Geometry check sheet. Reference: the model listing, model coordinates, mm. Round coordinates to 2 decimals unless told otherwise and drop trailing zeros. Loops run counter-clockwise (first coordinate to the right, second up) from the corner with the lowest first, then second, coordinate; pieces in that order, holes last. Notation, with made-up numbers: (74, 75.5) - (105, 75.5) arc R16 ccw to (105, 91.5) - close; hole circle Ø5 at (83.5, 35.5). An arc over 180 degrees is marked (long way). Answer in a Markdown table with one row per item. Add a question column.
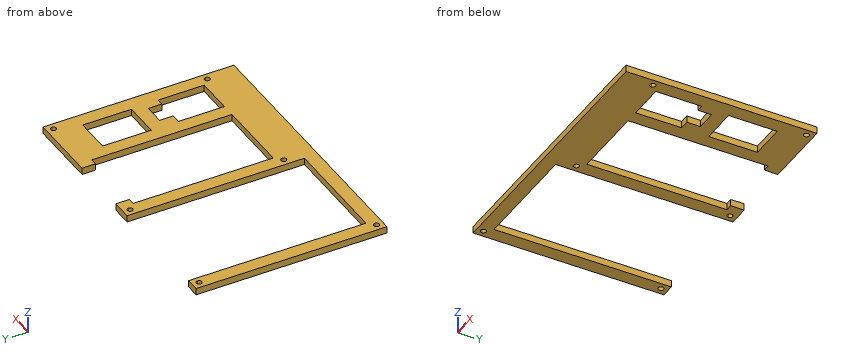
```python
from build123d import *

# Parameters (mm, degrees)
F1_DEPTH = 5


# Not quite as in the source:
# - a feature names something its author has since deleted; it is built from what else it names


with BuildPart() as f1:
    # F0 (on Top) → F1 (new body)
    with BuildSketch(Plane.XY):
        with BuildLine():
            Line((-134.3440142274, -1.256315279), (-139.3440142274, -1.256315279))
            Line((-139.3440142274, -1.256315279), (-139.3440142274, -6.256315279))
            Line((-139.3440142274, -6.256315279), (-136.3440142274, -6.256315279))
            ThreePointArc((-136.3440142274, -6.256315279), (-135.7582277898, -4.8421017166), (-134.3440142274, -4.256315279))
            Line((-134.3440142274, -4.256315279), (-134.3440142274, -1.256315279))
        make_face()
        with BuildLine():
            Line((-129.3440142274, -1.256315279), (-134.3440142274, -1.256315279))
            Line((-134.3440142274, -1.256315279), (-134.3440142274, -4.256315279))
            ThreePointArc((-134.3440142274, -4.256315279), (-132.929800665, -4.8421017166), (-132.3440142274, -6.256315279))
            ThreePointArc((-132.3440142274, -6.256315279), (-134.3440142274, -8.256315279), (-136.3440142274, -6.256315279))
            Line((-136.3440142274, -6.256315279), (-139.3440142274, -6.256315279))
            Line((-139.3440142274, -6.256315279), (-139.3440142274, -11.256315279))
            Line((-139.3440142274, -11.256315279), (-129.3440142274, -11.256315279))
            Line((-129.3440142274, -11.256315279), (-129.3440142274, -1.256315279))
        make_face()
        with BuildLine():
            Line((-221.3440142274, -6.256315279), (-221.3440142274, -1.256315279))
            Line((-221.3440142274, -1.256315279), (-231.3440142274, -1.256315279))
            Line((-231.3440142274, -1.256315279), (-231.3440142274, -132.256315279))
            Line((-231.3440142274, -132.256315279), (-221.3440142274, -132.256315279))
            Line((-221.3440142274, -132.256315279), (-221.3440142274, -128.856315279))
            Line((-221.3440142274, -128.856315279), (-221.3440142274, -14.656315279))
            Line((-221.3440142274, -14.656315279), (-221.3440142274, -11.256315279))
            Line((-221.3440142274, -11.256315279), (-226.3440142274, -11.256315279))
            Line((-226.3440142274, -11.256315279), (-226.3440142274, -8.256315279))
            ThreePointArc((-226.3440142274, -8.256315279), (-227.7582277898, -4.8421017166), (-224.3440142274, -6.256315279))
            Line((-224.3440142274, -6.256315279), (-221.3440142274, -6.256315279))
        make_face()
        Polygon((-124.3440142274, -1.256315279), (-129.3440142274, -1.256315279), (-129.3440142274, -11.256315279), (-126.5440142274, -11.256315279), (-126.3440142274, -11.256315279), (-124.3440142274, -11.256315279), align=None)
        Polygon((-129.3440142274, -11.256315279), (-139.3440142274, -11.256315279), (-139.3440142274, -14.656315279), (-139.3440142274, -114.756315279), (-129.3440142274, -114.756315279), (-129.3440142274, -111.756315279), (-129.3440142274, -108.756315279), (-129.3440142274, -27.956315279), (-129.3440142274, -27.456315279), (-129.3440142274, -14.056315279), align=None)
        with BuildLine():
            Line((-221.3440142274, -11.256315279), (-221.3440142274, -6.256315279))
            Line((-221.3440142274, -6.256315279), (-224.3440142274, -6.256315279))
            ThreePointArc((-224.3440142274, -6.256315279), (-224.929800665, -7.6705288414), (-226.3440142274, -8.256315279))
            Line((-226.3440142274, -8.256315279), (-226.3440142274, -11.256315279))
            Line((-226.3440142274, -11.256315279), (-221.3440142274, -11.256315279))
        make_face()
        with BuildLine():
            Line((-221.3440142274, -132.256315279), (-231.3440142274, -132.256315279))
            Line((-231.3440142274, -132.256315279), (-231.3440142274, -137.3912245035))
            Line((-231.3440142274, -137.3912245035), (-228.3440142274, -137.3912245035))
            ThreePointArc((-228.3440142274, -137.3912245035), (-226.3440142274, -135.3912245035), (-224.3440142274, -137.3912245035))
            ThreePointArc((-224.3440142274, -137.3912245035), (-224.929800665, -138.8054380659), (-226.3440142274, -139.3912245035))
            Line((-226.3440142274, -139.3912245035), (-226.3440142274, -142.256315279))
            Line((-226.3440142274, -142.256315279), (-221.3440142274, -142.256315279))
            Line((-221.3440142274, -142.256315279), (-221.3440142274, -132.256315279))
        make_face()
        with BuildLine():
            Line((-129.3440142274, -114.756315279), (-139.3440142274, -114.756315279))
            Line((-139.3440142274, -114.756315279), (-139.3440142274, -119.756315279))
            Line((-139.3440142274, -119.756315279), (-136.3440142274, -119.756315279))
            ThreePointArc((-136.3440142274, -119.756315279), (-134.3440142274, -117.756315279), (-132.3440142274, -119.756315279))
            ThreePointArc((-132.3440142274, -119.756315279), (-132.929800665, -121.1705288414), (-134.3440142274, -121.756315279))
            Line((-134.3440142274, -121.756315279), (-134.3440142274, -124.756315279))
            Line((-134.3440142274, -124.756315279), (-129.3440142274, -124.756315279))
            Line((-129.3440142274, -124.756315279), (-129.3440142274, -114.756315279))
        make_face()
        Polygon((-217.9440142274, -132.256315279), (-221.3440142274, -132.256315279), (-221.3440142274, -142.256315279), (-139.3440142274, -142.256315279), (-139.4949736476, -132.256315279), (-142.7440142274, -132.256315279), (-147.4240142274, -132.256315279), (-151.4240142274, -132.256315279), align=None)
        with BuildLine():
            Line((-228.3440142274, -137.3912245035), (-231.3440142274, -137.3912245035))
            Line((-231.3440142274, -137.3912245035), (-231.3440142274, -142.256315279))
            Line((-231.3440142274, -142.256315279), (-226.3440142274, -142.256315279))
            Line((-226.3440142274, -142.256315279), (-226.3440142274, -139.3912245035))
            ThreePointArc((-226.3440142274, -139.3912245035), (-227.7582277898, -138.8054380659), (-228.3440142274, -137.3912245035))
        make_face()
        with BuildLine():
            Line((-79.3440142274, -1.256315279), (-79.3440142274, -11.256315279))
            Line((-79.3440142274, -11.256315279), (-77.3440142274, -11.256315279))
            Line((-77.3440142274, -11.256315279), (-74.3440142274, -11.256315279))
            Line((-74.3440142274, -11.256315279), (-32.3440142274, -11.256315279))
            Line((-32.3440142274, -11.256315279), (-32.3440142274, -8.256315279))
            ThreePointArc((-32.3440142274, -8.256315279), (-33.7582277898, -4.8421017166), (-30.3440142274, -6.256315279))
            Line((-30.3440142274, -6.256315279), (-27.3440142274, -6.256315279))
            Line((-27.3440142274, -6.256315279), (-27.3440142274, -1.256315279))
            Line((-27.3440142274, -1.256315279), (-79.3440142274, -1.256315279))
        make_face()
        Polygon((-126.3440142274, -114.756315279), (-129.3440142274, -114.756315279), (-129.3440142274, -124.756315279), (-74.3440142274, -124.756315279), (-74.3440142274, -114.756315279), (-77.1940142274, -114.756315279), (-77.3440142274, -114.756315279), align=None)
        with BuildLine():
            Line((-136.3440142274, -119.756315279), (-139.3440142274, -119.756315279))
            Line((-139.3440142274, -119.756315279), (-139.3440142274, -124.756315279))
            Line((-139.3440142274, -124.756315279), (-139.1930548072, -124.756315279))
            Line((-139.1930548072, -124.756315279), (-134.3440142274, -124.756315279))
            Line((-134.3440142274, -124.756315279), (-134.3440142274, -121.756315279))
            ThreePointArc((-134.3440142274, -121.756315279), (-135.7582277898, -121.1705288414), (-136.3440142274, -119.756315279))
        make_face()
        Polygon((-139.3440142274, -132.256315279), (-139.4949736476, -132.256315279), (-139.3440142274, -142.256315279), (-129.3440142274, -142.256315279), (-129.3440142274, -124.756315279), (-134.3440142274, -124.756315279), (-139.1930548072, -124.756315279), (-139.3440142274, -124.756315279), (-139.3440142274, -128.856315279), align=None)
        Polygon((-74.3440142274, -124.756315279), (-129.3440142274, -124.756315279), (-129.3440142274, -142.256315279), (-77.3440142274, -142.256315279), (-74.3440142274, -142.256315279), align=None)
        Polygon((-32.3440142274, -11.256315279), (-74.3440142274, -11.256315279), (-74.3440142274, -14.256315279), (-74.3440142274, -26.056315279), (-74.3440142274, -103.156315279), (-74.3440142274, -111.906315279), (-74.3440142274, -114.756315279), (-64.3440142274, -114.756315279), (-64.3440142274, -105.506315279), (-64.3440142274, -82.706315279), (-64.3440142274, -80.756315279), (-64.3440142274, -60.756315279), (-64.3440142274, -59.006315279), (-64.3440142274, -26.456315279), (-64.3440142274, -24.756315279), (-62.6440142274, -24.756315279), (-39.5440142274, -24.756315279), (-37.8440142274, -24.756315279), (-27.3440142274, -24.756315279), (-27.3440142274, -14.656315279), (-27.3440142274, -11.256315279), align=None)
        with BuildLine():
            Line((-27.3440142274, -11.256315279), (-27.3440142274, -6.256315279))
            Line((-27.3440142274, -6.256315279), (-30.3440142274, -6.256315279))
            ThreePointArc((-30.3440142274, -6.256315279), (-30.929800665, -7.6705288414), (-32.3440142274, -8.256315279))
            Line((-32.3440142274, -8.256315279), (-32.3440142274, -11.256315279))
            Line((-32.3440142274, -11.256315279), (-27.3440142274, -11.256315279))
        make_face()
        Polygon((-74.3440142274, -114.756315279), (-74.3440142274, -124.756315279), (-37.3440142274, -124.756315279), (-37.3440142274, -119.756315279), (-37.3440142274, -114.756315279), (-39.2940142274, -114.756315279), (-62.3940142274, -114.756315279), (-64.3440142274, -114.756315279), align=None)
        Polygon((-37.3440142274, -124.756315279), (-74.3440142274, -124.756315279), (-74.3440142274, -142.256315279), (-27.3440142274, -142.256315279), (-27.3440142274, -124.756315279), (-32.3440142274, -124.756315279), align=None)
        with BuildLine():
            Line((-37.3440142274, -119.756315279), (-37.3440142274, -124.756315279))
            Line((-37.3440142274, -124.756315279), (-32.3440142274, -124.756315279))
            Line((-32.3440142274, -124.756315279), (-32.3440142274, -121.756315279))
            ThreePointArc((-32.3440142274, -121.756315279), (-33.7582277898, -121.1705288414), (-34.3440142274, -119.756315279))
            Line((-34.3440142274, -119.756315279), (-37.3440142274, -119.756315279))
        make_face()
        with BuildLine():
            Line((-32.3440142274, -121.756315279), (-32.3440142274, -124.756315279))
            Line((-32.3440142274, -124.756315279), (-27.3440142274, -124.756315279))
            Line((-27.3440142274, -124.756315279), (-27.3440142274, -114.756315279))
            Line((-27.3440142274, -114.756315279), (-37.3440142274, -114.756315279))
            Line((-37.3440142274, -114.756315279), (-37.3440142274, -119.756315279))
            Line((-37.3440142274, -119.756315279), (-34.3440142274, -119.756315279))
            ThreePointArc((-34.3440142274, -119.756315279), (-32.3440142274, -117.756315279), (-30.3440142274, -119.756315279))
            ThreePointArc((-30.3440142274, -119.756315279), (-30.929800665, -121.1705288414), (-32.3440142274, -121.756315279))
        make_face()
        Polygon((-27.3440142274, -114.756315279), (-27.3440142274, -24.756315279), (-37.8440142274, -24.756315279), (-37.8440142274, -26.456315279), (-37.8440142274, -59.006315279), (-37.8440142274, -60.756315279), (-39.5940142274, -60.756315279), (-62.5940142274, -60.756315279), (-64.3440142274, -60.756315279), (-64.3440142274, -80.756315279), (-62.3940142274, -80.756315279), (-57.3440142274, -80.756315279), (-57.3440142274, -70.756315279), (-42.3440142274, -70.756315279), (-42.3440142274, -80.756315279), (-39.2940142274, -80.756315279), (-37.3440142274, -80.756315279), (-37.3440142274, -82.706315279), (-37.3440142274, -105.506315279), (-37.3440142274, -114.756315279), align=None)
    extrude(amount=F1_DEPTH)


solid = f1.part
```
Q1. Cross-section at D-D, the plane x = -196. Enter the section's corners in (y, z).
Q2. Cross-section at B-B, the plane x = -40. Enter the section's corners in (y, z), plus the area to 3 significant figures.
Q3. Cross-section at C-C, the plane z = 3.9. State how many separate pieces and enclosed holes the cut face has, plus the area to 3 significant figures.
Q4. Depth check by flat-ended pin: P1, Ø10, axis at x = -145.5, y = -120, coming from the +Z side. Enter the tip coordinate at first touch or a pass-through.
Q5. Cross-section at A-A, the plane y = -15. Enter the section's corners in (x, z).
Q6. Scan lines: line 1 (X direction, y = -120, z = 3.1); line 2 (Y direction, x = -41, z = 2.1); line 3 (X direction, y = -12.5, z = 2.7). Record each from-to range of solid material in increasing order. Write a range as from..to.
Check sheet entries:
| question | item | result |
|---|---|---|
| 1 | outline | (-142.26, 0) - (-132.26, 0) - (-132.26, 5) - (-142.26, 5) - close |
| 2 | outline | (-142.26, 0) - (-114.76, 0) - (-114.76, 5) - (-142.26, 5) - close; (-80.76, 0) - (-60.76, 0) - (-60.76, 5) - (-80.76, 5) - close; (-24.76, 0) - (-1.26, 0) - (-1.26, 5) - (-24.76, 5) - close |
| 2 | area | 355 mm² |
| 3 | separate pieces | 1 |
| 3 | enclosed holes | 8 |
| 3 | area | 9,780 mm² |
| 4 | P1 | through |
| 5 | outline | (-231.34, 0) - (-221.34, 0) - (-221.34, 5) - (-231.34, 5) - close; (-139.34, 0) - (-129.34, 0) - (-129.34, 5) - (-139.34, 5) - close; (-74.34, 0) - (-27.34, 0) - (-27.34, 5) - (-74.34, 5) - close |
| 6 | line 1 | -231.34..-221.34, -139.34..-136.33, -132.36..-34.33, -30.36..-27.34 |
| 6 | line 2 | -142.26..-114.76, -80.76..-60.76, -24.76..-1.26 |
| 6 | line 3 | -231.34..-221.34, -139.34..-129.34, -74.34..-27.34 |
